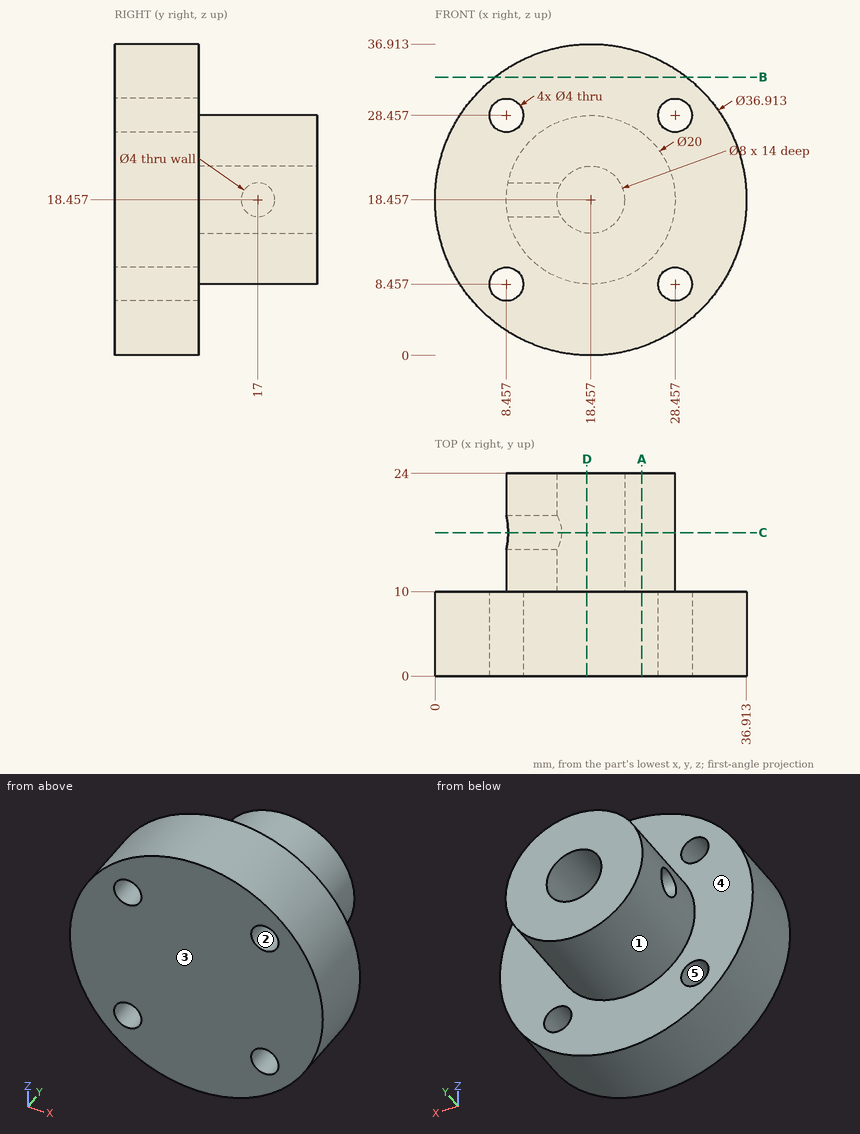
Can you work these out from the drawing? Everything is in mm from the part's minimum corner. A direction names the side the tool comes from. Give positions to 0.01 mm unless a question says otherwise; leave off trailing zeros. Order: outer loops, then holes, each group sorted by start corner. A loop starts at its lowest first (then second) coordinate and runs counter-clockwise, first axis right, second up.
1. We'd pull the mould along Z, two halves only. Please class the marked faces 1, 2 and 3: pulls with the +Z half, pulls with the -Z half, needs draft (parallel to the pull), parting line crosses it, or undercut.
2. Suppose I cut it at A-A (x = 24.5). List the corners of the cut face in (y, z) for me (1 decimal), plus the area to 3 significant figures.
3. Suppose I cut it at B-B (z = 33). List the corners of the cut face in (x, y) for me.
4. Suppose I cut it at D-D (x = 18). List the corners of the cut face in (y, z) for me (1 decimal).
5. For the marked faces 4 and 5, which set-ups out of +Z, -Z, +X, -X, +Y, -Y let a thin tool reach every point of the face, with its end or its side?
6. I need wall thicknesses on L1, parallel to Y at x = 33.5, z = 12.5; L2, parallel to Y at x = 14, z = 19 (1 decimal); L3, parallel to Z at x = 30, y = 3.5 (1 decimal). Which ranges of each line are inside material? Lowest first, please.
7. Will these pins go through, and if not, where does the flat tip stop? P1, Ø4.5, axis at y = 17, z = 18.46, coming from the +X side; P2, Ø8, axis at y = 13.5, z = 19, coming from the +X side; P3, Ø6, axis at x = 5, y = 8, coming from the -Z side; P4, Ø1, axis at x = 9.5, y = 17.5, coming from the -Z side.
8. Suppose I cut it at C-C (y = 17). List the corners of the cut face in (x, z) for me.
Solved:
1. face 1: parting line crosses it
1. face 2: undercut
1. face 3: needs draft
2. outline: (0, 1) - (10, 1) - (10, 10.5) - (24, 10.5) - (24, 26.4) - (10, 26.4) - (10, 35.9) - (0, 35.9) - close
2. area: 572 mm2
3. outline: (7.09, 0) - (29.82, 0) - (29.82, 10) - (7.09, 10) - close
4. outline: (0, 0) - (10, 0) - (10, 8.5) - (24, 8.5) - (24, 14.5) - (10, 14.5) - (10, 22.4) - (24, 22.4) - (24, 28.4) - (10, 28.4) - (10, 36.9) - (0, 36.9) - close
5. face 4: +Y
5. face 5: +Y, -Y
6. L1: y = 0 to 10
6. L2: y = 0 to 15.1, 18.9 to 24
6. L3: z = 4.1 to 7.2, 9.7 to 27.2, 29.7 to 32.9
7. P1: stops at x = 28.46
7. P2: stops at x = 36.91
7. P3: stops at z = 3.25
7. P4: stops at z = 13.12
8. outline: (8.66, 16.46) arc R10 ccw (long way) to (8.66, 20.46) - (14.99, 20.46) arc R4 cw (long way) to (14.99, 16.46) - close
